Part model, mm, in its own coordinate system. A direction names the side the tool comes from. Give positions to 0.01 mm unless a question says otherwise; leave off trailing zeros. Write each loop counter-clockwise with the first axis right and the second up, starting at its lowest first coordinate (ties: lowest second). Pieces come first, ordered by that corner, then holes.
```python
from build123d import *

# Parameters (mm, degrees)
PAD_DEPTH       = 6
SKETCH018_R     = 1.68
POCKET_DEPTH    = 6
SKETCH019_W     = 0.6
SKETCH019_H     = 7
POCKET001_DEPTH = 6
SKETCH020_W     = 1.2
SKETCH020_H     = 7
SKETCH020_W_2   = 1.51546
SKETCH020_W_3   = 1.6
POCKET002_DEPTH = 1.6
FILLET_R        = 2.2
FILLET001_R     = 3


with BuildPart() as part:
    # Sketch017 → Pad (new body)
    with BuildSketch(Plane(origin=(28, 46, 0), x_dir=(-1, 0, 0), z_dir=(0, 1, 0))):
        Polygon((-14.4, 32), (-14.4, 14), (-12, 14), (-12, 0), (0, 0), (0, 18), (-2.4, 18), (-2.4, 32), align=None)
    extrude(amount=PAD_DEPTH)

    # Sketch018 → Pocket (cut)
    with BuildSketch(Plane(origin=(28, 52, 0), x_dir=(-1, 0, 0), z_dir=(0, 1, 0))):
        with Locations((-7.3, 3.9)):
            Circle(SKETCH018_R)
        with Locations((-7.3, 16)):
            Circle(SKETCH018_R)
        with Locations((-7.3, 28.1)):
            Circle(SKETCH018_R)
    extrude(amount=-POCKET_DEPTH, mode=Mode.SUBTRACT)

    # Sketch019 → Pocket001 (cut)
    with BuildSketch(Plane(origin=(28, 52, 0), x_dir=(-1, 0, 0), z_dir=(0, 1, 0))):
        with Locations((-0.3, 9.5)):
            Rectangle(SKETCH019_W, SKETCH019_H)
        with Locations((-14.1, 22.3)):
            Rectangle(SKETCH019_W, SKETCH019_H)
    extrude(amount=-POCKET001_DEPTH, mode=Mode.SUBTRACT)

    # Sketch020 → Pocket002 (cut)
    with BuildSketch(Plane(origin=(28, 46, 0), x_dir=(-1, 0, 0), z_dir=(0, -1, 0))):
        with Locations((-7.2, -9.5)):
            Rectangle(SKETCH020_W, SKETCH020_H)
        with Locations((-5.2, -9.5)):
            Rectangle(SKETCH020_W, SKETCH020_H)
        with Locations((-3.2, -9.5)):
            Rectangle(SKETCH020_W, SKETCH020_H)
        with Locations((-1.2, -9.5)):
            Rectangle(SKETCH020_W, SKETCH020_H)
        with Locations((-11.35773, -9.5)):
            Rectangle(SKETCH020_W_2, SKETCH020_H)
        with Locations((-9.2, -9.5)):
            Rectangle(SKETCH020_W, SKETCH020_H)
        with Locations((-13.4, -22.3)):
            Rectangle(SKETCH020_W, SKETCH020_H)
        with Locations((-11.4, -22.3)):
            Rectangle(SKETCH020_W, SKETCH020_H)
        with Locations((-9.4, -22.3)):
            Rectangle(SKETCH020_W, SKETCH020_H)
        with Locations((-7.4, -22.3)):
            Rectangle(SKETCH020_W, SKETCH020_H)
        with Locations((-5.4, -22.3)):
            Rectangle(SKETCH020_W, SKETCH020_H)
        with Locations((-3.2, -22.3)):
            Rectangle(SKETCH020_W_3, SKETCH020_H)
    extrude(amount=-POCKET002_DEPTH, mode=Mode.SUBTRACT)

    # Fillet
    fillet_edges = [part.edges().sort_by_distance(p)[0] for p in [
        (40, 49, 14),
        (30.4, 49, 18),
    ]]
    fillet(fillet_edges, radius=FILLET_R)

    # Fillet001
    fillet001_edges = [part.edges().sort_by_distance(p)[0] for p in [
        (30.4, 49, 32),
        (42.4, 49, 32),
        (28, 49, 0),
        (40, 49, 0),
    ]]
    fillet(fillet001_edges, radius=FILLET001_R)


solid = part.part
```
1) Saw through at A-A, the plane z = 16. Write the cut outline in (x, y).
Answers follow:
outline: (28, 46) - (33.62, 46) - (33.62, 52) - (28, 52) - close; (36.98, 46) - (42.4, 46) - (42.4, 52) - (36.98, 52) - close
2) Saw through at C-C, the plane y = 51.6. Write the cut outline in (x, z), then the cut area to 3 significant figures.
Answers follow:
outline: (28, 3) arc R3 ccw to (31, 0) - (37, 0) arc R3 ccw to (40, 3) - (40, 11.8) arc R2.2 cw to (42.2, 14) - (42.4, 14) - (42.4, 18.8) - (41.8, 18.8) - (41.8, 25.8) - (42.4, 25.8) - (42.4, 29) arc R3 ccw to (39.4, 32) - (33.4, 32) arc R3 ccw to (30.4, 29) - (30.4, 20.2) arc R2.2 cw to (28.2, 18) - (28, 18) - (28, 13) - (28.6, 13) - (28.6, 6) - (28, 6) - close; hole circle Ø3.36 at (35.3, 3.9); hole circle Ø3.36 at (35.3, 16); hole circle Ø3.36 at (35.3, 28.1)
area: 353 mm2
3) 3-axis set-ups, long thin cutter, end or side, ignore diameter. For faces 1 (the face through (37, 47.6, 9)), 2 (the face through (29.77, 49.04, 18.66)), 3 (the face through (39, 47, 6)), 4 (the face through (28.3, 48.4, 13)), 5 (the face through (42.4, 49, 27)): which of +Z, -Z, +X, -X, +Y, -Y reach the whole face in a straight line?
Answers follow:
face 1: -Y
face 2: +Z, -X, +Y, -Y
face 3: +X, -Y
face 4: -X, -Y
face 5: +Z, -Z, +X, +Y, -Y
4) Pin check, flat tips, straight feed: pin 1 Ø0.8 at (x, z) = (41, 21.5) entering from -Y; pin 2 Ø1.8 at (x, y) = (42, 49) entering from -Z; pin 3 Ø1.5 at (y, z) = (51, 8) entering from -X; pin 4 Ø1.8 at (y, z) = (46.5, 23.5) entering from -X. Stop position of each tip, or through.
Answers follow:
pin 1: stops at y = 46
pin 2: stops at z = 13.71
pin 3: stops at x = 28.6
pin 4: stops at x = 32
5) Saw through at D-D, the plane z = 3.9. Write the cut outline in (x, y), then the cut area to 3 significant figures.
Answers follow:
outline: (28, 46) - (33.62, 46) - (33.62, 52) - (28, 52) - close; (36.98, 46) - (40, 46) - (40, 52) - (36.98, 52) - close
area: 51.8 mm2
6) Saw through at B-B, the plane x = 35.3. Write the cut outline in (y, z), then the cut area to 3 significant figures.
Answers follow:
outline: (46, 0) - (52, 0) - (52, 2.22) - (46, 2.22) - close; (46, 5.58) - (52, 5.58) - (52, 14.32) - (46, 14.32) - (46, 13) - (47.6, 13) - (47.6, 6) - (46, 6) - close; (46, 17.68) - (52, 17.68) - (52, 26.42) - (46, 26.42) - (46, 25.8) - (47.6, 25.8) - (47.6, 18.8) - (46, 18.8) - close; (46, 29.78) - (52, 29.78) - (52, 32) - (46, 32) - close
area: 109 mm2
7) Two-plate mould, pull along Z, no slides. Class faces 6 (the face through (30.6, 47, 10)), 7 (the face through (28, 49, 4)), 8 (the face through (39.1, 49.04, 0.86)): +Z half, -Z half, draft (parallel to the pull), parting line (faces both ways), or undercut.
Answers follow:
face 6: undercut
face 7: draft
face 8: -Z half
8) Wall check: L1, parallel to Z at x = 35.3, y = 49.2; L2, parallel to Z at x = 35.3, y = 47.45; L3, parallel to X at y = 46.3, z = 20.5. Give the ranges that are in metal, low to high.
Answers follow:
L1: z = 0 to 2.22, 5.58 to 14.32, 17.68 to 26.42, 29.78 to 32
L2: z = 0 to 2.22, 5.58 to 6, 13 to 14.32, 17.68 to 18.8, 25.8 to 26.42, 29.78 to 32
L3: x = 32 to 32.8, 34 to 34.8, 36 to 36.8, 38 to 38.8, 40 to 40.8
